```python
from build123d import *

# Parameters (mm, degrees)
SKETCH2_W               = 48.26
SKETCH2_H               = 83.82
SKETCH2_R               = 1.27
BOSS_EXTRUDE1_DEPTH     = 1.524
SKETCH3_R               = 1.27
BOSS_EXTRUDE2_DEPTH     = 1.524
MIRROR2_COPY_1_SKETCH_R = 1.27
MIRROR2_COPY_1_DEPTH    = 1.524
CUT_EXTRUDE1_DEPTH      = 1.524
MIRROR4_COPY_1_DEPTH    = 1.524
FILLET1_R               = 1.5875


with BuildPart() as part:
    # Sketch2 → Boss-Extrude1 (new body)
    with BuildSketch(Plane(origin=(0, 0, 0), x_dir=(1, 0, 0), z_dir=(0, 1, 0))):
        with Locations((0, -100.64115)):
            Rectangle(SKETCH2_W, SKETCH2_H)
        with Locations(Location((20.955, -140.6398, 0), (0, 0, 90))):
            Circle(SKETCH2_R, mode=Mode.SUBTRACT)
        with Locations(Location((-20.955, -140.6398, 0), (0, 0, 90))):
            Circle(SKETCH2_R, mode=Mode.SUBTRACT)
        with Locations(Location((20.955, -60.6425, 0), (0, 0, 90))):
            Circle(SKETCH2_R, mode=Mode.SUBTRACT)
        with Locations(Location((-20.955, -60.6425, 0), (0, 0, 90))):
            Circle(SKETCH2_R, mode=Mode.SUBTRACT)
    extrude(amount=BOSS_EXTRUDE1_DEPTH)

    # Sketch3 → Boss-Extrude2 (add, through all)
    with BuildSketch(Plane(origin=(0, 0, 0), x_dir=(1, 0, 0), z_dir=(0, 1, 0))):
        Polygon((-2.921, -67.681554482), (23.533261314, -52.408179591), (29.375261314, -62.526820409), (2.921, -77.8001953), align=None)
        with Locations(Location((20.955, -60.6425, 0), (0, 0, 90))):
            Circle(SKETCH3_R, mode=Mode.SUBTRACT)
    boss_extrude2 = extrude(amount=BOSS_EXTRUDE2_DEPTH)

    # Mirror1: Boss-Extrude2 across plane
    add(boss_extrude2.mirror(Plane.XY.offset(100.64115)))

    # Mirror2: Boss-Extrude2 across plane
    add(boss_extrude2.mirror(Plane(origin=(0, 0, 0), x_dir=(0, 0, 1), z_dir=(1, 0, 0))))

    # Mirror2 copy 1 sketch → Mirror2 copy 1 (add, through all)
    with BuildSketch(Plane(origin=(0, 0, 201.2823), x_dir=(-1, 0, 0), z_dir=(0, 1, 0))):
        Polygon((-2.921, -67.681554482), (23.533261314, -52.408179591), (29.375261314, -62.526820409), (2.921, -77.8001953), align=None)
        with Locations(Location((20.955, -60.6425, 0), (0, 0, 90))):
            Circle(MIRROR2_COPY_1_SKETCH_R, mode=Mode.SUBTRACT)
    extrude(amount=MIRROR2_COPY_1_DEPTH)

    # Sketch4 → Cut-Extrude1 (cut)
    with BuildSketch(Plane(origin=(0, 1.524, 0), x_dir=(1, 0, 0), z_dir=(0, 1, 0))):
        Polygon((4.0259, -77.162280987), (4.0259, -94.60865), (18.034, -94.60865), (18.034, -69.074700682), align=None)
        Polygon((4.0259, -64.82715), (4.0259, -70.416520442), (13.706973588, -64.82715), align=None)
        Polygon((4.0259, -64.82715), (0, -64.82715), (0, -72.740874891), (4.0259, -70.416520442), align=None)
    cut_extrude1 = extrude(amount=-CUT_EXTRUDE1_DEPTH, mode=Mode.SUBTRACT)

    # Mirror3: Cut-Extrude1 across plane
    add(cut_extrude1.mirror(Plane(origin=(0, 0, 0), x_dir=(0, 0, 1), z_dir=(1, 0, 0))), mode=Mode.SUBTRACT)

    # Mirror4: Cut-Extrude1 across plane
    add(cut_extrude1.mirror(Plane.XY.offset(100.64115)), mode=Mode.SUBTRACT)

    # Mirror4 copy 1 sketch → Mirror4 copy 1 (cut)
    with BuildSketch(Plane(origin=(0, 1.524, 201.2823), x_dir=(-1, 0, 0), z_dir=(0, 1, 0))):
        Polygon((4.0259, -77.162280987), (4.0259, -94.60865), (18.034, -94.60865), (18.034, -69.074700682), align=None)
        Polygon((4.0259, -64.82715), (4.0259, -70.416520442), (13.706973588, -64.82715), align=None)
        Polygon((4.0259, -64.82715), (0, -64.82715), (0, -72.740874891), (4.0259, -70.416520442), align=None)
    extrude(amount=-MIRROR4_COPY_1_DEPTH, mode=Mode.SUBTRACT)

    # Fillet1
    fillet1_edges = [part.edges().sort_by_distance(p)[0] for p in [
        (-29.375261314, 0.762, 138.755479591),
        (18.034, 0.762, 69.074700682),
        (18.034, 0.762, 94.60865),
        (4.0259, 0.762, 94.60865),
        (4.0259, 0.762, 77.162280987),
        (13.706973588, 0.762, 64.82715),
        (0, 0.762, 72.740874891),
        (-18.034, 0.762, 94.60865),
        (-18.034, 0.762, 69.074700682),
        (-4.0259, 0.762, 77.162280987),
        (-4.0259, 0.762, 94.60865),
        (-13.706973588, 0.762, 64.82715),
        (-18.034, 0.762, 132.207599318),
        (-18.034, 0.762, 106.67365),
        (-4.0259, 0.762, 106.67365),
        (-4.0259, 0.762, 124.120019013),
        (-13.706973588, 0.762, 136.45515),
        (0, 0.762, 128.541425109),
        (18.034, 0.762, 106.67365),
        (18.034, 0.762, 132.207599318),
        (4.0259, 0.762, 124.120019013),
        (4.0259, 0.762, 106.67365),
        (13.706973588, 0.762, 136.45515),
        (24.13, 0.762, 65.555173441),
        (12.581555311, 0.762, 58.73115),
        (29.375261314, 0.762, 62.526820409),
        (23.533261314, 0.762, 52.408179591),
        (12.581555311, 0.762, 142.55115),
        (23.533261314, 0.762, 148.874120409),
        (24.13, 0.762, 135.727126559),
        (29.375261314, 0.762, 138.755479591),
        (-29.375261314, 0.762, 62.526820409),
        (-12.581555311, 0.762, 58.73115),
        (-23.533261314, 0.762, 52.408179591),
        (-24.13, 0.762, 65.555173441),
        (-24.13, 0.762, 135.727126559),
        (-12.581555311, 0.762, 142.55115),
        (-23.533261314, 0.762, 148.874120409),
    ]]
    fillet(fillet1_edges, radius=FILLET1_R)


solid = part.part
```
Could you check a few things on this model? Use its own coordinates, in mm. A direction names the side the tool comes from. Coordinates: 2 decimals unless noted, no trailing zeros. Order: outer loops, then holes, each group sorted by start corner. A loop starts at its lowest first (then second) coordinate and runs counter-clockwise, first axis right, second up. Notation, with made-up numbers: M 61.25,-16.5 L 82.25,-16.5 A26 ccw 82.25,17.5 Z; hole C -23,-34.75 d10. An arc over 180 degrees is marked long. Use one line per item in the form item = value. Start each with the question number.
1. Please list where these lines run through material, in increasing order: line 1 (X direction, y = 1, z = 108); line 2 (X direction, y = 1.15, z = 127); line 3 (Z direction, x = -10, y = 0.2).
2. Suppose I cut it at A-A on z = 121. Write out the boundary of the cut face in (x, y), then the cut area to 3 significant figures.
3. Suppose I cut it at B-B on y = 1.25. Count the separate pieces of the cut face and the enclosed holes in it, then the cut area to 3 significant figures.
4. For pin 1 (1 mm diameter, centred on x = -3, z = 70.5, fed in from +Y); pin 2 (0.5 mm diameter, centred on y = 1, z = 115.5, fed in from +X); pin 3 (0.8 mm diameter, centred on x = 5.5, y = 0.5, fed in from -Z); pin 4 (0.8 mm diameter, centred on y = 0.5, z = 121.5, fed in from -X), each with a flat end and sliding along its axis, tell me the tip position at first contact or that it passes through.
5. On a 3-axis mill with a long thin cutter (end or side, diameter ignored), from which of +Z, -Z, +X, -X, +Y, -Y can I reach the whole of each face in a straight line? I mean faces 1 (the flat face through (26.484, 0.751, 137.086)), 2 (the flat face through (17.49, 0.751, 145.385)), 3 (the flat face through (10.312, 0.773, 73.533)). Say none if no direction works.
6. We'd pull the mould along Z, two halves only. Please class faces 4 (the flat face through (26.424, 0.751, 57.416)), 5 (the flat face through (-10.312, 0.773, 73.533)), 6 (the flat face through (-26.424, 0.751, 143.866)): +Z half, -Z half, draft (parallel to the pull), parting line (faces both ways), or undercut.
7. Suppose I cut it at C-C on z = 105. Write out the boundary of the cut face in (x, y).
Geometry says:
q1.line_1 = -24.13 to -18.01, -4.05 to 4.05, 18.01 to 24.13
q1.line_2 = -24.13 to -18.03, -9.01 to 9.01, 18.03 to 24.13
q1.line_3 = 58.73 to 73.71, 94.61 to 106.67, 127.57 to 142.55
q2.outline = M -24.13,0 L -18.03,0 L -18.03,1.52 L -24.13,1.52 Z; M -4.03,0 L 4.03,0 L 4.03,1.52 L -4.03,1.52 Z; M 18.03,0 L 24.13,0 L 24.13,1.52 L 18.03,1.52 Z
q2.area = 30.9 mm^2
q3.separate_pieces = 1
q3.enclosed_holes = 10
q3.area = 2,920 mm^2
q4.pin_1 = 1.52
q4.pin_2 = 24.13
q4.pin_3 = 58.73
q4.pin_4 = -24.13
q5.face_1 = +X, +Y, -Y
q5.face_2 = +Z, +Y, -Y
q5.face_3 = +Y, -Y
q6.face_4 = -Z half
q6.face_5 = undercut
q6.face_6 = +Z half
q7.outline = M -24.13,0 L 24.13,0 L 24.13,1.52 L -24.13,1.52 Z
